```python
from build123d import *

# Parameters (mm, degrees)
F0_W      = 25
F0_H      = 40
F0_R      = 6.25
F1_DEPTH  = 3.2
F2_W      = 25
F2_H      = 40
F3_DEPTH  = 40
F4_W      = 15
F4_H      = 46.4
F4_R      = 2.25
F5_DEPTH  = 5
F6_SIZE   = 2
F7_R      = 2.25
F8_DEPTH  = 3.2
F9_W      = 46.4
F9_H      = 70
F10_DEPTH = 36.8
F11_W     = 25
F11_H     = 40
F11_R     = 6.25
F12_DEPTH = 3.2
F13_R     = 7.5
F14_DEPTH = 4


with BuildPart() as f1:
    # F0 (on Top) → F1 (new body)
    with BuildSketch(Plane.XY):
        Rectangle(F0_W, F0_H)
        Circle(F0_R, mode=Mode.SUBTRACT)
    extrude(amount=F1_DEPTH)

    # F2 (on face) → F3 (join)
    with BuildSketch(Plane.XY.offset(3.2)):
        with BuildLine():
            Line((15.7, -23.2), (15.7, 23.2))
            Line((15.7, 23.2), (7.5, 23.2))
            Line((7.5, 23.2), (7.5, 27.5))
            ThreePointArc((7.5, 27.5), (0, 35), (-7.5, 27.5))
            Line((-7.5, 27.5), (-7.5, 23.2))
            Line((-7.5, 23.2), (-15.7, 23.2))
            Line((-15.7, 23.2), (-15.7, -23.2))
            Line((-15.7, -23.2), (-7.5, -23.2))
            Line((-7.5, -23.2), (-7.5, -27.5))
            ThreePointArc((-7.5, -27.5), (0, -35), (7.5, -27.5))
            Line((7.5, -27.5), (7.5, -23.2))
            Line((7.5, -23.2), (15.7, -23.2))
        make_face()
        Polygon((-3.4352341017, -27.5), (-1.7176170508, -24.525), (1.7176170508, -24.525), (3.4352341017, -27.5), (1.7176170508, -30.475), (-1.7176170508, -30.475), align=None, mode=Mode.SUBTRACT)
        Rectangle(F2_W, F2_H, mode=Mode.SUBTRACT)
        Polygon((-3.4352341017, 27.5), (-1.7176170508, 30.475), (1.7176170508, 30.475), (3.4352341017, 27.5), (1.7176170508, 24.525), (-1.7176170508, 24.525), align=None, mode=Mode.SUBTRACT)
    extrude(amount=-F3_DEPTH)

    # F4 (on face) → F5 (join)
    with BuildSketch(Plane.XY.offset(3.2)):
        with Locations((-23.2, 0)):
            Rectangle(F4_W, F4_H)
        with Locations((-23.2, -13.2)):
            Circle(F4_R, mode=Mode.SUBTRACT)
        with Locations((-23.2, 13.2)):
            Circle(F4_R, mode=Mode.SUBTRACT)
    extrude(amount=-F5_DEPTH)

    # F6
    f6_edges = [f1.edges().sort_by_distance(p)[0] for p in [
        (15.7, 23.2, -16.8),
        (-15.7, 23.2, -19.3),
        (-15.7, -23.2, -19.3),
        (15.7, -23.2, -16.8),
        (-30.7, 23.2, 0.7),
        (-30.7, -23.2, 0.7),
    ]]
    chamfer(f6_edges, length=F6_SIZE)

    # F7 (on face) → F8 (join)
    with BuildSketch(Plane(origin=(0, 0, -36.8), x_dir=(1, 0, 0), z_dir=(0, 0, -1))):
        Polygon((1.7176170508, 30.475), (-1.7176170508, 30.475), (-3.4352341017, 27.5), (-1.7176170508, 24.525), (1.7176170508, 24.525), (3.4352341017, 27.5), align=None)
        with Locations((0, 27.5)):
            Circle(F7_R, mode=Mode.SUBTRACT)
        Polygon((-3.4352341017, -27.5), (-1.7176170508, -30.475), (1.7176170508, -30.475), (3.4352341017, -27.5), (1.7176170508, -24.525), (-1.7176170508, -24.525), align=None)
        with Locations((0, -27.5)):
            Circle(F7_R, mode=Mode.SUBTRACT)
    extrude(amount=-F8_DEPTH)

    # F9 (on face) → F10 (cut)
    with BuildSketch(Plane.XY.offset(3.2)):
        with Locations((-7.5, 0)):
            Rectangle(F9_W, F9_H)
    extrude(amount=-F10_DEPTH, mode=Mode.SUBTRACT)

    # F11 (on face) → F12 (join)
    with BuildSketch(Plane.XY.offset(-33.6)):
        Rectangle(F11_W, F11_H)
        Circle(F11_R, mode=Mode.SUBTRACT)
    extrude(amount=-F12_DEPTH)

    # F13 (on face) → F14 (join)
    with BuildSketch(Plane.XY.offset(-33.6)):
        with Locations((0, 27.5)):
            Circle(F13_R)
        Polygon((-3.4352341017, 27.5), (-1.7176170508, 30.475), (1.7176170508, 30.475), (3.4352341017, 27.5), (1.7176170508, 24.525), (-1.7176170508, 24.525), align=None, mode=Mode.SUBTRACT)
        with Locations((0, -27.5)):
            Circle(F13_R)
        Polygon((-3.4352341017, -27.5), (-1.7176170508, -24.525), (1.7176170508, -24.525), (3.4352341017, -27.5), (1.7176170508, -30.475), (-1.7176170508, -30.475), align=None, mode=Mode.SUBTRACT)
    extrude(amount=F14_DEPTH)


solid = f1.part
```
CAD build for the part. Positions are in the model's coordinates, mm. A direction names the side the tool comes from. Give positions to 0.01 mm unless a question says otherwise; leave off trailing zeros. Order: outer loops, then holes, each group sorted by start corner. A loop starts at its lowest first (then second) coordinate and runs counter-clockwise, first axis right, second up. Notation, with made-up numbers: M 85.5,9.5 L 116.5,9.5 A6 ccw 116.5,17.5 Z; hole C 45.25,53 d10. An arc over 180 degrees is marked long. Put each result on its own line as item: value. Start each with the question number.
(1) Saw through at C-C, the plane y = 0. Write the cut outline in (x, z).
(2) Flat gauge pins, fed straight in: pin 1 Ø1 at (y, z) = (24.5, -35) entering from -X; pin 2 Ø3 at (x, y) = (0.5, -28.5) entering from +Z; pin 3 Ø1.6 at (x, z) = (-12, -34.5) entering from +Y; pin 4 Ø7.5 at (x, y) = (0, 0) entering from -Z. Where does each tip first touch, or does it go through?
(3) Saw through at B-B, the plane x = 0. Write the cut outline in (y, z) (3 decimals).
(4) Saw through at A-A, the plane z = -32.25. Write the cut outline in (x, y) (3 decimals).
(5) Mould opens along X. For faces 1 (the flat face through (14.7, -22.2, -35.2)), 2 (the flat face through (2, 26, -33.6)), 3 (the flat face through (0, 24, -29.6)), 4 (the flat face through (-7.5, -25, -35)) say: +X half, -X half, draft (parallel to the pull), parting line (faces both ways), or undercut.
(6) Saw through at D-D, the plane y = -15.5. Write the cut outline in (x, z).
(7) Drill centre lines: line 1 along Y through (x, z) = (0, -34.35); line 2 along X through (y, z) = (27.5, -35.2); line 3 along Y through (x, z) = (-1, -31) (3 decimals). Where is each one in solid material? Low to high.
(8) Which spindle directions (+Z, -Z, +X, -X, +Y, -Y) get a long thin tool onto all of the face, cutting with end or side? Do faces 5 (the flat face through (-11, -23.2, -35)), 6 (the flat face through (-11, 23.2, -35)), 7 (the flat face through (0, -7, -36.8)), 8 (the flat face through (2, -29, -33.6)). Say none if no direction does.
Check result:
1. outline: M -15.7,-36.8 L -6.25,-36.8 L -6.25,-33.6 L -15.7,-33.6 Z; M 6.25,-36.8 L 15.7,-36.8 L 15.7,-33.6 L 6.25,-33.6 Z
2. pin 1: stops at x = -7.5
2. pin 2: stops at z = -33.6
2. pin 3: stops at y = 23.2
2. pin 4: passes through
3. outline: M -35,-36.8 L -29.75,-36.8 L -29.75,-33.6 L -30.475,-33.6 L -30.475,-29.6 L -35,-29.6 Z; M -25.25,-36.8 L -6.25,-36.8 L -6.25,-33.6 L -20,-33.6 L -20,-29.6 L -24.525,-29.6 L -24.525,-33.6 L -25.25,-33.6 Z; M 6.25,-36.8 L 25.25,-36.8 L 25.25,-33.6 L 24.525,-33.6 L 24.525,-29.6 L 20,-29.6 L 20,-33.6 L 6.25,-33.6 Z; M 29.75,-36.8 L 35,-36.8 L 35,-29.6 L 30.475,-29.6 L 30.475,-33.6 L 29.75,-33.6 Z
4. outline: C 0,-27.5 d15; C 0,27.5 d15; hole M -3.435,-27.5 L -1.718,-30.475 L 1.718,-30.475 L 3.435,-27.5 L 1.718,-24.525 L -1.718,-24.525 Z; hole M -3.435,27.5 L -1.718,24.525 L 1.718,24.525 L 3.435,27.5 L 1.718,30.475 L -1.718,30.475 Z
5. face 1: +X half
5. face 2: undercut
5. face 3: draft
5. face 4: -X half
6. outline: M -15.7,-36.8 L 15.7,-36.8 L 15.7,-33.6 L -15.7,-33.6 Z
7. line 1: y = -35 to -29.75, -25.25 to -6.25, 6.25 to 25.25, 29.75 to 35
7. line 2: x = -7.5 to -2.25, 2.25 to 7.5
7. line 3: y = -34.933 to -30.475, -24.525 to -20.067, 20.067 to 24.525, 30.475 to 34.933
8. face 5: +Z, -Z, -X, -Y
8. face 6: +Z, -Z, -X, +Y
8. face 7: -Z, +X, -X, +Y, -Y
8. face 8: +Z
